Could you check a few things on this drawing? It's one solid part, dimensions in mm from its lowest x, y, z. A direction names the side the tool comes from. Give positions to 0.01 mm unless a question says otherwise; leave off trailing zeros. Loops run counter-clockwise (first coordinate to the right, second up) from the corner with the lowest first, then second, coordinate; pieces in that order, holes last. Notation, with made-up numbers: (-3, -19.75) - (30, -19.75) arc R19 cw to (30, 14.25) - close; hole circle Ø9 at (74, 18). An arc over 180 degrees is marked (long way). Write item = value, one per line.
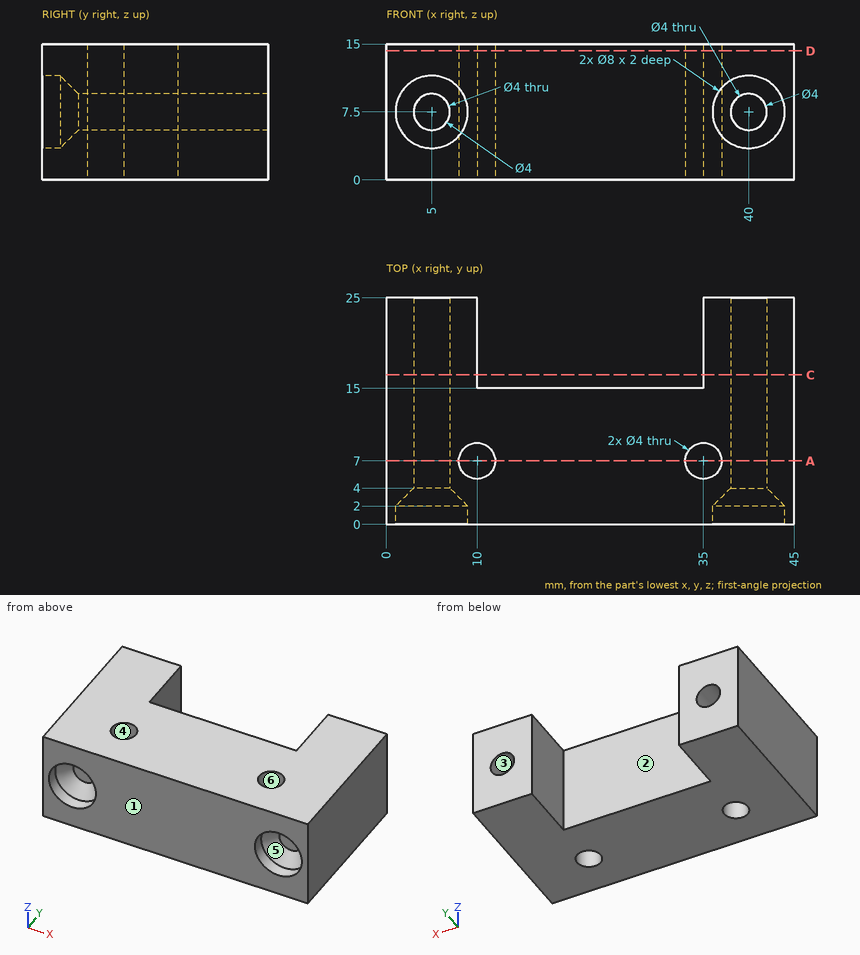
Q1. For pin 1 (3 mm diameter, centred on x = 10, y = 7, fed in from +Z); pin 2 (6.5 mm diameter, centred on x = 40, z = 7.5, fed in from -Y), each with a flat end and sliding along its axis, tell me the tip position at first contact or that it passes through.
Output:
pin_1 = through
pin_2 = 2.75
Q2. I need wall thicknesses on L1, parallel to X at y = 19, z = 7.5; L2, parallel to X at y = 7, z = 10.75; L3, parallel to X at y = 4, z = 7.75 (1 decimal). Which ranges of each line are inside material? Lowest first, please.
Output:
L1 = 0 to 3, 7 to 10, 35 to 38, 42 to 45
L2 = 0 to 8, 12 to 33, 37 to 45
L3 = 0 to 3, 7 to 38, 42 to 45
Q3. Imagine slicing it at C-C, the plane y = 16.5. Write out the boundary of the cut face in (x, z), then the cut area to 3 significant figures.
Output:
outline = (0, 0) - (10, 0) - (10, 15) - (0, 15) - close; (35, 0) - (45, 0) - (45, 15) - (35, 15) - close; hole circle Ø4 at (5, 7.5); hole circle Ø4 at (40, 7.5)
area = 275 mm2
Q4. Which directions (+Z, -Z, +X, -X, +Y, -Y) give clear straight access to the entire face, cutting with the end or side of a thin tool? Please do the marked faces 1 and 2.
Output:
face_1 = +Z, -Z, +X, -X, -Y
face_2 = +Z, -Z, +Y
Q5. We'd pull the mould along Y, two halves only. Please class the marked faces 3, 4, 5 and 6: released by +Y, released by -Y, zero draft, split by the parting line, or undercut.
Output:
face_3 = zero draft
face_4 = undercut
face_5 = released by -Y
face_6 = undercut
Q6. Imagine slicing it at A-A, the plane y = 7. Write out the boundary of the cut face in (x, z).
Output:
outline = (0, 0) - (8, 0) - (8, 15) - (0, 15) - close; (12, 0) - (33, 0) - (33, 15) - (12, 15) - close; (37, 0) - (45, 0) - (45, 15) - (37, 15) - close; hole circle Ø4 at (5, 7.5); hole circle Ø4 at (40, 7.5)
Q7. Imagine slicing it at D-D, the plane z = 14.25. Write out the boundary of the cut face in (x, y).
Output:
outline = (0, 0) - (45, 0) - (45, 25) - (35, 25) - (35, 15) - (10, 15) - (10, 25) - (0, 25) - close; hole circle Ø4 at (10, 7); hole circle Ø4 at (35, 7)
